from build123d import *

# Parameters (mm, degrees)
F2_R     = 5.26415
F3_DEPTH = 25.4
F5_R     = 2.54
F6_R     = 2.54


with BuildPart() as f1:
    # F0 (on Front) → F1 (revolve)
    with BuildSketch(Plane.XZ):
        Polygon((-229.616, 0), (0, 0), (0, 19.05), (-23.876, 19.05), (-33.311927, 25.20315), (-199.136, 25.20315), (-199.136, 34.98215), (-209.296, 34.98215), (-219.456, 25.20315), (-229.616, 25.20315), align=None)
    revolve(axis=Axis((-114.808, 0, 0), (-1, 0, 0)))

    # F2 (on face) → F3 (cut)
    with BuildSketch(Plane(origin=(-229.616, 0, 0), x_dir=(0, -1, 0), z_dir=(-1, 0, 0))):
        Circle(F2_R)
    extrude(amount=-F3_DEPTH, mode=Mode.SUBTRACT)

    # F5
    f5_edges = [f1.edges().sort_by_distance(p)[0] for p in [
        (-23.876, 0, -19.05),
        (-33.311927, 0, -25.20315),
    ]]
    fillet(f5_edges, radius=F5_R)

    # F6
    f6_edges = [f1.edges().sort_by_distance(p)[0] for p in [
        (-199.136, 0, -25.20315),
    ]]
    fillet(f6_edges, radius=F6_R)


solid = f1.part
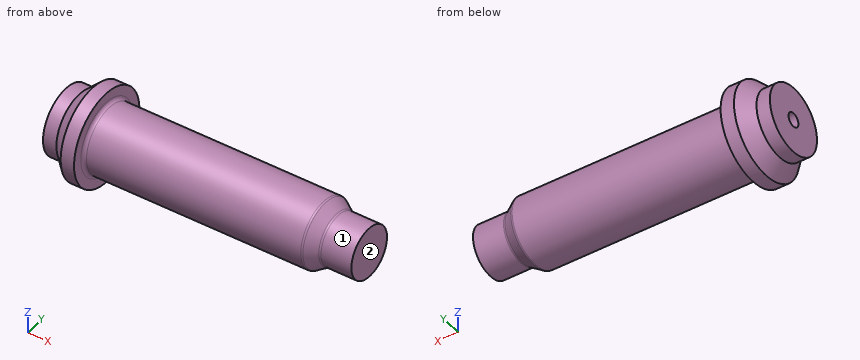
Can you work these out from the model? Positions are in its coordinate system, mm. Face numbers are marked on the shaded views. A direction names the side the tool comes from. Round coordinates to 2 decimals unless told otherwise and drop trailing zeros. Write each loop counter-clockwise with the first axis right and the second up, starting at its lowest first coordinate (ties: lowest second). Pieces come first, ordered by that corner, then holes. Notation, with made-up numbers: (25.5, 4) -> (82.5, 4) arc R28 cw to (82.5, 41) -> close; hole circle Ø3 at (41, 76.5). An arc over 180 degrees is marked (long way). Use one line per item in the form item = value. Start each with the question number.
Q1. Which directions (+Z, -Z, +X, -X, +Y, -Y) give clear straight access to the entire face, cutting with the end or side of a thin tool? Please do the marked faces 1 and 2.
Q2. Imagine slicing it at B-B (x = -131.5). Please give me the cut outline in (y, z), then the cut area to 3 significant figures.
Q3. I'm going to push flat-ended pins straight in: P1, Ø6, axis at x = -177, z = 18.5, coming from the -Y side; P2, Ø12, axis at x = -86.5, y = 23, coming from the -Z side; P3, Ø1, axis at x = -152.5, y = -4, coming from the +Z side. Where does each tip first touch, or does it pass through?
Q4. If I drill on probe 1 along X at (y, z) = (-2.5, 2.5); probe 2 along Y at (x, z) = (-50, 0.5); probe 3 along Z at (x, y) = (-216, 0), over which ranges is the centre line in solid material (lowest first)? Write a range as [from, to].
Q5. Imagine slicing it at A-A (x = -20). Please give me the cut outline in (y, z), then the cut area to 3 significant figures.
Worked out:
q1.face_1 = +X
q1.face_2 = +Z, -Z, +X, +Y, -Y
q2.outline = circle Ø50.41 at (0, 0)
q2.area = 2,000 mm^2
q3.P1 = -19.87
q3.P2 = -18.61
q3.P3 = 24.96
q4.probe_1 = [-204.22, 0]
q4.probe_2 = [-25.2, 25.2]
q4.probe_3 = [-28.53, -5.26], [5.26, 28.53]
q5.outline = circle Ø38.1 at (0, 0)
q5.area = 1,140 mm^2
